Autodesk Inventor part; units mm, degrees
ref_plane "YZ Plane" through (0, 0, 0) normal (1, 0, 0) x (0, 1, 0)
ref_plane "XZ Plane" through (0, 0, 0) normal (0, 1, 0) x (-1, 0, 0)
ref_plane "XY Plane" through (0, 0, 0) normal (0, 0, 1) x (1, 0, 0)
sketch "Sketch1" plane through (0, 0, 0) normal (0, 1, 0) x (-1, 0, 0)
  line L0 (-20, 80) -> (20, 80)
  line L1 (20, 80) -> (20, -80)
  line L2 (20, -80) -> (-20, -80)
  line L3 (-20, -80) -> (-20, 80)
  line L4 (-20, 80) -> (20, -80) construction
  line L5 (20, 80) -> (-20, -80) construction
  line L6 (20, 80) -> (30, 80)
  line L7 (30, 80) -> (30, -80)
  line L8 (30, -80) -> (20, -80)
  line L9 (20, -80) -> (20, 80)
  line L10 (-20, 80) -> (-30, 80)
  line L11 (-30, 80) -> (-30, -80)
  line L12 (-30, -80) -> (-20, -80)
  line L13 (-20, -80) -> (-20, 80)
  circle A0 centre (30, 80) radius 1.5
  circle A1 centre (20, 80) radius 1.5
  circle A2 centre (-20, 80) radius 1.5
  circle A3 centre (-30, 80) radius 1.5
  circle A4 centre (30, -80) radius 1.5
  circle A5 centre (-30, -80) radius 1.5
  line L14 (-85.15, 40) -> (85.15, 40)
  line L15 (85.15, 40) -> (85.15, -40)
  line L16 (85.15, -40) -> (-85.15, -40)
  line L17 (-85.15, -40) -> (-85.15, 40)
  line L18 (-85.15, 40) -> (85.15, -40) construction
  line L19 (85.15, 40) -> (-85.15, -40) construction
  line L20 (85.15, 40) -> (-85.15, 40)
  line L21 (-85.15, 40) -> (-85.15, 50)
  line L22 (-85.15, 50) -> (85.15, 50)
  line L23 (85.15, 50) -> (85.15, 40)
  line L24 (85.15, -40) -> (-85.15, -40)
  line L25 (-85.15, -40) -> (-85.15, -50)
  line L26 (-85.15, -50) -> (85.15, -50)
  line L27 (85.15, -50) -> (85.15, -40)
  circle A6 centre (-85.15, 50) radius 1.5
  circle A7 centre (-85.15, 40) radius 1.5
  circle A8 centre (-85.15, -40) radius 1.5
  circle A9 centre (-85.15, -50) radius 1.5
  circle A10 centre (-20, -80) radius 1.5
  circle A11 centre (20, -80) radius 1.5
  circle A12 centre (85.15, -40) radius 1.5
  circle A13 centre (85.15, -50) radius 1.5
  circle A14 centre (85.15, 50) radius 1.5
  circle A15 centre (85.15, 40.1297) radius 1.5
  line L28 (85.15, 50) -> (-85.15, 50)
  line L29 (-85.15, 50) -> (-85.15, 53.5)
  line L30 (-85.15, 53.5) -> (85.15, 53.5)
  line L31 (85.15, 53.5) -> (85.15, 50)
  line L32 (-30, 80) -> (-33.5, 80)
  line L33 (-33.5, 80) -> (-33.5, -80)
  line L34 (-33.5, -80) -> (-30, -80)
  line L35 (-30, -80) -> (-30, 80)
  line L36 (85.15, -50) -> (-85.15, -50)
  line L37 (-85.15, -50) -> (-85.15, -53.5)
  line L38 (-85.15, -53.5) -> (85.15, -53.5)
  line L39 (85.15, -53.5) -> (85.15, -50)
  line L40 (30, -80) -> (-33.5, -80)
  line L41 (-33.5, -80) -> (-33.5, -83)
  line L42 (-33.5, -83) -> (30, -83)
  line L43 (30, -83) -> (30, -80)
  line L44 (30, 80) -> (33.5, 80)
  line L45 (33.5, 80) -> (33.5, -83)
  line L46 (33.5, -83) -> (30, -83)
  line L47 (30, -83) -> (30, 80)
  line L48 (33.5, 80) -> (-33.5, 80)
  line L49 (-33.5, 80) -> (-33.5, 83)
  line L50 (-33.5, 83) -> (33.5, 83)
  line L51 (33.5, 83) -> (33.5, 80)
  line L52 (85.15, 53.5) -> (88.15, 53.5)
  line L53 (88.15, 53.5) -> (88.15, -53.5)
  line L54 (88.15, -53.5) -> (85.15, -53.5)
  line L55 (85.15, -53.5) -> (85.15, 53.5)
  line L56 (-85.15, 53.5) -> (-88.15, 53.5)
  line L57 (-88.15, 53.5) -> (-88.15, -53.5)
  line L58 (-88.15, -53.5) -> (-85.15, -53.5)
  line L59 (-85.15, -53.5) -> (-85.15, 53.5)
  point P0 (0, 0)
  point P1 (-33.5, 53.5)
  point P2 (-33.5, -53.5)
  point P3 (33.5, -53.5)
  point P4 (33.5, 53.5)
  point P5 (-18.5, 80)
  point P6 (-20, 78.5)
  point P7 (20, 78.5)
  point P8 (18.5, 80)
  dimension "d0" = 40
  dimension "d1" = 160
  dimension "d2" = 10
  dimension "d3" = 10
  dimension "d4" = 3
  dimension "d5" = 3
  dimension "d6" = 3
  dimension "d7" = 3
  dimension "d8" = 3
  dimension "d9" = 3
  dimension "d10" = 170.3
  dimension "d11" = 80
  dimension "d12" = 10
  dimension "d13" = 10
  dimension "d14" = 3
  dimension "d15" = 3
  dimension "d16" = 3
  dimension "d17" = 3
  dimension "d18" = 3
  dimension "d19" = 3
  dimension "d20" = 3
  dimension "d21" = 3
  dimension "d22" = 3
  dimension "d23" = 3
  dimension "d24" = 3.5
  dimension "d25" = 3.5
  dimension "d26" = 3.5
  dimension "d27" = 3
  dimension "d28" = 3.5
  dimension "d29" = 3
  dimension "d30" = 3
  dimension "d31" = 3
extrude "Extrusion1" add sketch "Sketch1" along normal blind 3 contours A2 L10 A3 L32 L49 L50 L51 L44 A0 L6 A1 L0 | L0 A1 L1 L30 L3 A2 | L3 L30 L11 A3 L10 A2 | L30 L1 L22 L3 | L3 L22 L11 L30 | L6 A0 L7 L30 L1 A1 | L22 L1 L14 L3 | L3 L14 L11 L22 | L30 L33 L32 A3 L11 | L11 L22 L33 L30 | L30 L7 L22 L1 | L14 L1 L16 L3 | L3 L16 L11 L14 | L11 L14 L33 L22 | L22 L7 L14 L1 | L33 L22 A6 L29 L30 | L30 L45 L22 L7 | L7 A0 L44 L45 L30 | L16 L1 L26 L3 | L3 L26 L11 L16 | L11 L16 L33 L14 | L14 L7 L16 L1 | L33 L14 A7 L21 A6 L22 | L22 L45 L14 L7 | L29 A6 L21 A7 L17 A8 L25 A9 L37 L58 L57 L56 | L30 L31 A14 L22 L45 | L26 L1 L38 L3 | L3 L38 L11 L26 | L16 L7 L26 L1 | L11 L26 L33 L16 | L33 L16 A8 L17 A7 L14 | L14 L45 L16 L7 | L22 A14 L23 A15 L14 L45 | L52 L53 L54 L39 A13 L27 A12 L15 A15 L23 A14 L31 | L38 L1 A11 L2 A10 L3 | L3 A10 L12 A5 L11 L38 | L11 L38 L33 L26 | L26 L7 L38 L1 | L16 L45 L26 L7 | L33 L26 A9 L25 A8 L16 | L14 A15 L15 A12 L16 L45 | L11 A5 L34 L33 L38 | L38 L7 A4 L8 A11 L1 | L33 L38 L37 A9 L26 | L26 L45 L38 L7 | L16 A12 L27 A13 L26 L45 | L2 A11 L8 A4 L43 L42 L41 L34 A5 L12 A10 | L38 L45 L46 L43 A4 L7 | L26 A13 L39 L38 L45
fillet "Fillet1" radius 5 4 edges at (33.5, 1.5, 53.5) (-33.5, 1.5, 53.5) (-33.5, 1.5, -53.5) (33.5, 1.5, -53.5)
fillet "Fillet2" radius 3 8 edges at (-88.15, 1.5, 53.5) (-88.15, 1.5, -53.5) (-33.5, 1.5, -83) (33.5, 1.5, -83) (88.15, 1.5, -53.5) (88.15, 1.5, 53.5) (33.5, 1.5, 83) (-33.5, 1.5, 83)
sketch "Sketch2" plane through (0, 3, 0) normal (0, 1, 0) x (1, 0, 0)
  line L0 (88.15, -50.5) -> (88.15, 50.5)
  line L1 (88.15, 0) -> (73.15, 0)
  line L2 (73.15, 0) -> (73.15, -10)
  line L3 (73.15, -10) -> (88.15, -10)
  line L4 (88.15, -10) -> (88.15, 0)
  line L5 (73.15, 0) -> (88.15, 0)
  line L6 (88.15, 0) -> (88.15, 10)
  line L7 (88.15, 10) -> (73.15, 10)
  line L8 (73.15, 10) -> (73.15, 0)
  point P0 (0, 0)
  dimension "d36" = 15
  dimension "d37" = 10
  dimension "d38" = 10
extrude "Extrusion2" cut sketch "Sketch2" against normal blind 3
fillet "Fillet3" radius 3 4 edges at (73.15, 1.5, -10) (88.15, 1.5, -10) (73.15, 1.5, 10) (88.15, 1.5, 10)
properties part number "cover"
Geometry check sheet. Reference: the model listing, model coordinates, mm. Round coordinates to 2 decimals unless told otherwise and drop trailing zeros. Order: outer loops, then holes, each group sorted by start corner. A loop starts at its lowest first (then second) coordinate and runs counter-clockwise, first axis right, second up. Notation, with made-up numbers: M 69.25,-13 L 96.25,-13 A19 ccw 96.25,-8 Z; hole C 12.5,65 d4. An arc over 180 degrees is marked long. Write each question's results on one line, items separated by ' | '. Start each with the question number.
1. Go/stop test with flat-tipped pins: P1, Ø1.5, axis at y = 1.5, z = 70.5, coming from the +X side; P2, Ø1.5, axis at y = 1, z = -69.5, coming from the -X side. Record where each tip stops, or that it passes through.
2. Cross-section at A-A on x = 56. Record the boundary of the cut face in (y, z).
3. Draft check along Y on faces 1 (the face through (1, 3, 1)), 2 (the face through (-35, 1.52, -54.93)), 3 (the face through (1, 0, 1)). Enter one of: pulls with the +Y half, pulls with the -Y half, needs draft (parallel to the pull), parting line crosses it, or undercut.
4. Material ranges on L1, parallel to X at y = 1.75, z = -50; L2, parallel to X at y = 1.75, z = 80; L3, parallel to Z at x = -30, y = 2.2, recorded low to high. Write a range as from..to.
5. Cross-section at B-B on y = 1.3. Give the number of separate pieces and of enclosed holes in the cut face, plus the area to 3 significant figures.
Resolved:
1) P1: x = 33.5 | P2: x = -33.5
2) outline: M 0,-53.5 L 3,-53.5 L 3,53.5 L 0,53.5 Z
3) face 1: pulls with the +Y half | face 2: needs draft | face 3: pulls with the -Y half
4) L1: -88.15..-86.65, -83.65..83.65, 86.65..88.15 | L2: -33.5..-31.5, -28.5..-21.5, -18.5..18.5, 21.5..28.5, 31.5..33.5 | L3: -83..-81.5, -78.5..78.5, 81.5..83
5) separate pieces: 1 | enclosed holes: 16 | area: 22,400 mm2
